Read the model definition and answer for the solid it produces. Units are mm, in the model's axes. Face numbers are marked on the shaded views. A direction names the side the tool comes from. Coordinates: 2 decimals unless noted, no trailing zeros. Write each loop counter-clockwise with the first axis right and the second up, starting at its lowest first coordinate (ties: lowest second). Pieces come first, ordered by that corner, then holes. Notation, with made-up numbers: (-27, 66) -> (-5, 66) arc R18 ccw to (-5, 101) -> close; hole circle Ø8 at (-24, 31). An arc over 180 degrees is marked (long way). Answer as a JSON object with one key per item and string values. Group by question number.
(1) For a pull along Y with two mould halves and no side action, classify the marked faces 4, 5 and 6 as +Y half, -Y half, draft (parallel to the pull), parting line (faces both ways), or undercut.
(2) Find section A-A (x = 0). Give the vertices of the cut face in (y, z).
(3) Straight lines are drawn through the part: L1, parallel to X at y = 0, z = 81.75; L2, parallel to Y at x = 0, z = 83; L3, parallel to Y at x = -3, z = 53.5. For each, find the intervals that lie inside material, in ascending order.
(4) Which of the six approach directions +Z, -Z, +X, -X, +Y, -Y give full straight-line access (tool end or side, diameter ignored) to the marked faces 1, 2 and 3?
(5) Find section B-B (y = 0). Give the vertices of the cut face in (x, z).
(6) Find section D-D (x = 23). Give the vertices of the cut face in (y, z).
(7) Flat-ended cylindrical pins translate along their axes: P1, Ø2, axis at y = 2.5, z = 57.5, coming from the -X side; P2, Ø16.5, axis at x = 11.5, z = 45, coming from the -Y side. Find the tip coordinate at first contact, or state that the pin passes through.
(8) Find section C-C (z = 61). Give the vertices of the cut face in (x, y).
from build123d import *

# Parameters (mm, degrees)
F0_W     = 97.3299
F0_H     = 81.834436
F1_DEPTH = 101.6
F2_R     = 19.644425
F3_DEPTH = 25.4
F5_R     = 12.777111
F6_DEPTH = 25.4
F4_R     = 28.866366
F7_DEPTH = 25.4


with BuildPart() as f1:
    # F0 (on Top) → F1 (new body)
    with BuildSketch(Plane.XY):
        Rectangle(F0_W, F0_H)
    extrude(amount=F1_DEPTH)

    # F2 (on face) → F3 (cut)
    with BuildSketch(Plane.XY.offset(101.6)):
        Circle(F2_R)
    extrude(amount=-F3_DEPTH, mode=Mode.SUBTRACT)

    # F5 (on face) → F6 (cut)
    with BuildSketch(Plane(origin=(-48.66495, 0, 0), x_dir=(0, -1, 0), z_dir=(-1, 0, 0))):
        with Locations((0, 56.615394)):
            Circle(F5_R)
    extrude(amount=-F6_DEPTH, mode=Mode.SUBTRACT)

    # F4 (on face) → F7 (cut)
    with BuildSketch(Plane.XZ.offset(40.917218)):
        with Locations((-0.084508, 51.481884)):
            Circle(F4_R)
    extrude(amount=-F7_DEPTH, mode=Mode.SUBTRACT)


solid = f1.part
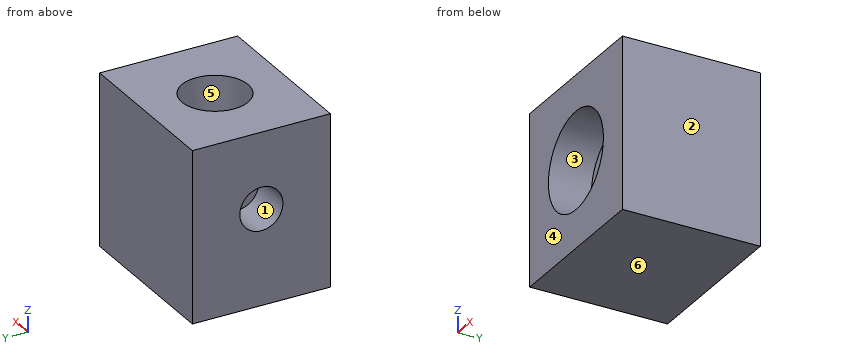
Results below:
{
 "1": {"face 4": "-Y half", "face 5": "undercut", "face 6": "draft"},
 "2": {"outline": "(-40.92, 0) -> (40.92, 0) -> (40.92, 101.6) -> (19.64, 101.6) -> (19.64, 76.2) -> (-15.52, 76.2) -> (-15.52, 22.62) -> (-40.92, 22.62) -> close; (-40.92, 80.35) -> (-19.64, 80.35) -> (-19.64, 101.6) -> (-40.92, 101.6) -> close"},
 "3": {"L1": "x = -48.66 to -19.64, 19.64 to 48.66", "L2": "y = -40.92 to -19.64, 19.64 to 40.92", "L3": "y = -15.52 to 40.92"},
 "4": {"face 1": "-X", "face 2": "+Z, -Z, +X, +Y, -Y", "face 3": "-Y"},
 "5": {"outline": "(-48.66, 0) -> (48.66, 0) -> (48.66, 101.6) -> (19.64, 101.6) -> (19.64, 76.2) -> (-19.64, 76.2) -> (-19.64, 101.6) -> (-48.66, 101.6) -> (-48.66, 69.39) -> (-23.26, 69.39) -> (-23.26, 43.84) -> (-48.66, 43.84) -> close"},
 "6": {"outline": "(-40.92, 0) -> (40.92, 0) -> (40.92, 101.6) -> (-40.92, 101.6) -> (-40.92, 68.81) -> (-15.52, 68.81) -> (-15.52, 34.15) -> (-40.92, 34.15) -> close"},
 "7": {"P1": "stops at x = -23.26", "P2": "stops at y = -15.52"},
 "8": {"outline": "(-48.66, -40.92) -> (-27.34, -40.92) -> (-27.34, -15.52) -> (27.17, -15.52) -> (27.17, -40.92) -> (48.66, -40.92) -> (48.66, 40.92) -> (-48.66, 40.92) -> (-48.66, 12) -> (-23.26, 12) -> (-23.26, -12) -> (-48.66, -12) -> close"}
}
